The model under review builds one solid part; all positions refer to its coordinate system, in mm. Face numbers are marked on the shaded views. A direction names the side the tool comes from. Coordinates: 2 decimals unless noted, no trailing zeros. Loops run counter-clockwise (first coordinate to the right, second up) from the corner with the lowest first, then second, coordinate; pieces in that order, holes last. Notation, with made-up numbers: (36, 59.25) - (61, 59.25) arc R23 ccw to (61, 77.25) - close; hole circle Ø9 at (46.25, -28). An arc over 180 degrees is marked (long way). Answer in a Markdown table with one row per item. Add a question column.
(1) We need section A-A on x = 0. Write out the cut boundary in (y, z).
(2) For P1, Ø5.5, axis at x = -3.5, z = 2, coming from the -Y side; P2, Ø17.5, axis at x = -6.5, y = 10, coming from the +Z side; P3, Ø1, axis at x = 2, z = -11.5, coming from the +Y side; P4, Ø5.5, axis at y = 26, z = 3.5, coming from the +X side, all flat-tipped, find the tip position at first contact; note any pin that passes through.
(3) Machinability: for the marked faces 1 and 2, which of the approach directions +Z, -Z, +X, -X, +Y, -Y give a long, thin tool a straight path to every point of the face, cutting with its end or side? Answer none if there is none.
(4) For line 1 along X through (y, z) = (28.5, 1.5); line 2 along Z through (x, y) = (-4.5, 18); line 3 along Y through (x, z) = (17.5, -11), list the stretches that pass through material, from the lowest coordinate up.
from build123d import *

# Parameters (mm, degrees)
Y_KSEKLIK_EKSTR_ZYON1_DEPTH      = 20
Y_KSEKLIK_EKSTR_ZYON1_DEPTH_BACK = 20
Y_KSEKLIK_EKSTR_ZYON2_DEPTH      = 5
RADYUS1_R                        = 2
RADYUS2_R                        = 2


with BuildPart() as part:
    # Çizim1 → Yükseklik-Ekstrüzyon1 (new, two sides: drawn at the far end of the back side and taken through both)
    with BuildSketch(Plane(origin=(0, 0, 0), x_dir=(0, 0, -1), z_dir=(1, 0, 0)).offset(-Y_KSEKLIK_EKSTR_ZYON1_DEPTH_BACK)):
        Polygon((0, 0), (40, 0), (0, 40), align=None)
    extrude(amount=Y_KSEKLIK_EKSTR_ZYON1_DEPTH + Y_KSEKLIK_EKSTR_ZYON1_DEPTH_BACK)

    # Çizim3 → Yükseklik-Ekstrüzyon2 (add)
    with BuildSketch(Plane.XY):
        Polygon((-13.028588348, 32.028588348), (-12.028588348, 33.028588348), (12.028588348, 33.028588348), (13.028588348, 32.028588348), (13.028588348, 20.827816013), (12.028588348, 19.827816013), (-12.028588348, 19.827816013), (-13.028588348, 20.827816013), align=None)
    extrude(amount=Y_KSEKLIK_EKSTR_ZYON2_DEPTH)

    # Radyus1
    radyus1_edges = [part.edges().sort_by_distance(p)[0] for p in [
        (20, 20, 0),
        (20, 20, -20),
        (-20, 20, -20),
        (-20, 20, 0),
    ]]
    fillet(radyus1_edges, radius=RADYUS1_R)

    # Radyus2
    # the kernel refuses this fillet: 2 mm, written as the material it takes off along each edge
    with BuildSketch(Plane(origin=(18, 35.171572875, -2), x_dir=(0, 0, 1), z_dir=(1, 0, 0))) as radyus2_piece_1_section:
        Polygon((0, 0), (RADYUS2_R, 0), (RADYUS2_R, -RADYUS2_R * 2.41421356237), (-RADYUS2_R * 0.707106781187, -RADYUS2_R * 0.707106781187), align=None)
    radyus2_piece_1 = extrude(amount=RADYUS2_R, mode=Mode.PRIVATE)
    radyus2_piece_1 = radyus2_piece_1 - Plane(origin=(18, 35.171572875, -2), x_dir=(0, -0.9238795325112866, -0.38268343236508967), z_dir=(1, 0, 0)) * Sphere(RADYUS2_R, mode=Mode.PRIVATE)
    add(radyus2_piece_1, mode=Mode.SUBTRACT)
    with BuildSketch(Plane(origin=(-18, 35.171572875, -2), x_dir=(0, 0, 1), z_dir=(-1, 0, 0))) as radyus2_piece_2_section:
        Polygon((0, 0), (RADYUS2_R, 0), (RADYUS2_R, RADYUS2_R * 2.41421356237), (-RADYUS2_R * 0.707106781187, RADYUS2_R * 0.707106781187), align=None)
    radyus2_piece_2 = extrude(amount=RADYUS2_R, mode=Mode.PRIVATE)
    radyus2_piece_2 = radyus2_piece_2 - Plane(origin=(-18, 35.171572875, -2), x_dir=(0, -0.9238795325112866, -0.38268343236508967), z_dir=(-1, 0, 0)) * Sphere(RADYUS2_R, mode=Mode.PRIVATE)
    add(radyus2_piece_2, mode=Mode.SUBTRACT)
    with BuildSketch(Plane(origin=(18, 40, 0), x_dir=(0, -1, 0), z_dir=(-1, 0, 0))) as radyus2_piece_3:
        with BuildLine():
            CenterArc((RADYUS2_R * 2.41421356237, -RADYUS2_R), RADYUS2_R, 90, 135)
            Line((RADYUS2_R * 1.70710678119, -RADYUS2_R * 1.70710678119), (0, 0))
            Line((0, 0), (RADYUS2_R * 2.41421356237, 0))
        make_face()
    extrude(amount=36, mode=Mode.SUBTRACT)


solid = part.part
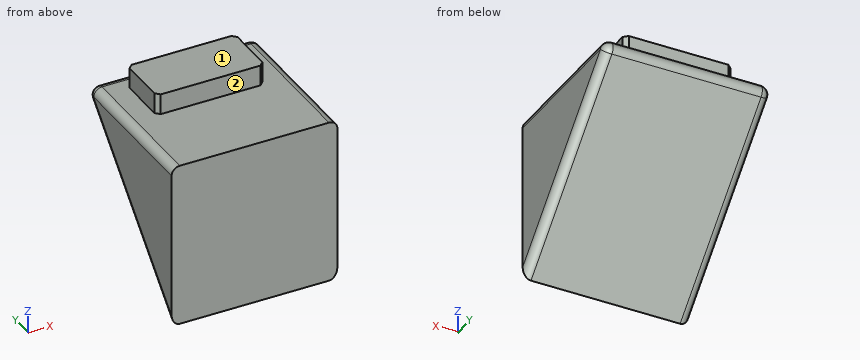
Outcome:
| question | item | result |
|---|---|---|
| 1 | outline | (0, -40) - (36.59, -3.41) arc R2 ccw to (35.17, 0) - (33.03, 0) - (33.03, 5) - (19.83, 5) - (19.83, 0) - (0, 0) - close |
| 2 | P1 | y = 0 |
| 2 | P2 | z = 0 |
| 2 | P3 | y = 29 |
| 2 | P4 | x = 13.03 |
| 3 | face 1 | +Z, +X, -X, +Y, -Y |
| 3 | face 2 | +Z, +X, -X, -Y |
| 4 | line 1 | -13.03 to 13.03 |
| 4 | line 2 | -22 to 0 |
| 4 | line 3 | 0 to 29 |
